from build123d import *

# Parameters (mm, degrees)
SKETCH1_R               = 13.365
BOSS_EXTRUDE1_DEPTH     = 10
SKETCH2_R               = 15
BOSS_EXTRUDE2_DEPTH     = 2
BOSS_EXTRUDE3_START     = -2
SKETCH3_R               = 15
BOSS_EXTRUDE3_DEPTH     = 2
CUT_EXTRUDE1_DEPTH      = 10
CUT_EXTRUDE1_DEPTH_BACK = 24.452078799
SKETCH4_R               = 5
SKETCH4_R_2             = 2.5


with BuildPart() as part:
    # Sketch1 → Boss-Extrude1 (new body)
    with BuildSketch(Plane(origin=(0, 0, 0), x_dir=(1, 0, 0), z_dir=(0, 1, 0))):
        with Locations(Location((0, 0, 0), (0, 0, 270))):
            Circle(SKETCH1_R)
    extrude(amount=BOSS_EXTRUDE1_DEPTH)

    # Sketch2 → Boss-Extrude2 (add)
    with BuildSketch(Plane(origin=(0, 10, 0), x_dir=(1, 0, 0), z_dir=(0, 1, 0))):
        with Locations(Location((0, 0, 0), (0, 0, 270))):
            Circle(SKETCH2_R)
    extrude(amount=-BOSS_EXTRUDE2_DEPTH)

    # Sketch3 → Boss-Extrude3 (add)
    with BuildSketch(Plane.XZ.offset(BOSS_EXTRUDE3_START)):
        with Locations(Location((0, 0, 0), (0, 0, 90))):
            Circle(SKETCH3_R)
    extrude(amount=BOSS_EXTRUDE3_DEPTH)

    # Sketch4 → Cut-Extrude1 (cut, two sides: drawn at the far end of the back side and taken through both)
    with BuildSketch(Plane.XZ.offset(-CUT_EXTRUDE1_DEPTH_BACK)):
        with Locations(Location((0, 0, 0), (0, 0, 90))):
            Circle(SKETCH4_R)
        with Locations(Location((0, 9, 0), (0, 0, 90))):
            Circle(SKETCH4_R_2)
        with Locations(Location((9, 0, 0), (0, 0, 90))):
            Circle(SKETCH4_R_2)
        with Locations(Location((0, -9, 0), (0, 0, 90))):
            Circle(SKETCH4_R_2)
        with Locations(Location((-9, 0, 0), (0, 0, 90))):
            Circle(SKETCH4_R_2)
    extrude(amount=CUT_EXTRUDE1_DEPTH + CUT_EXTRUDE1_DEPTH_BACK, mode=Mode.SUBTRACT)


solid = part.part
CAD build for the part. Positions are in the model's coordinates, mm. A direction names the side the tool comes from. Round coordinates to 2 decimals unless told otherwise and drop trailing zeros. Write each loop counter-clockwise with the first axis right and the second up, starting at its lowest first coordinate (ties: lowest second). Pieces come first, ordered by that corner, then holes. Notation, with made-up numbers: M 87,42 L 113,42 A14 cw 113,46 Z; hole C 63,61.25 d8. An arc over 180 degrees is marked long. Use a Markdown table: item, result. Add a question column.
1. 3-axis set-ups, long thin cutter, end or side, ignore diameter. For faces 1 (the face through (-4, 0, -4)), 2 (the face through (2.2, 2, -13.4)): which of +Z, -Z, +X, -X, +Y, -Y reach the whole face in a straight line?
2. Drill centre lines: probe 1 along X at (y, z) = (5.5, 0) (3 decimals); probe 2 along Z at (x, y) = (1.25, 1.5); probe 3 along Y at (x, z) = (-4.25, -13.5). Where is each one in solid material? Low to high.
3. Flat gauge pins, fed straight in: P1, Ø5, axis at y = 1.5, z = 4.5, coming from the -X side; P2, Ø4.5, axis at x = 9, z = 0, coming from the -Y side; P3, Ø4, axis at y = 4.5, z = -9.5, coming from the +X side; P4, Ø6, axis at y = 3, z = 4, coming from the -X side. Where does each tip first touch, or does it go through?
4. Slice it at A-A on z = 0. Give the cut face in (x, y) (3 decimals), then the cut area to 3 significant figures.
5. Slice it at D-D on x = -10.25. Give the cut face in (y, z).
6. Slice it at B-B on x = 0. Give the cut face in (y, z) (3 decimals), then the cut area to 3 significant figures.
7. Slice it at C-C on y = 1.25. Give the cut face in (x, z), then the cut area to 3 significant figures.
8. Pull direction X, two halves, no side cores. Call faces 3 (the face through (11.44, 5.07, -0.54)), 4 (the face through (0.66, 9.014, -14.985)), 5 (the face through (4, 10, -4)): released by +X, released by -X, zero draft, split by the parting line, or undercut.
Reply:
| question | item | result |
|---|---|---|
| 1 | face 1 | +Z, -Z, +X, -X, -Y |
| 1 | face 2 | none |
| 2 | probe 1 | x = -13.365 to -11.5, -6.5 to -5, 5 to 6.5, 11.5 to 13.365 |
| 2 | probe 2 | z = -14.95 to -11.17, -6.83 to -4.84, 4.84 to 6.83, 11.17 to 14.95 |
| 2 | probe 3 | y = 0 to 2, 8 to 10 |
| 3 | P1 | stops at x = -14.87 |
| 3 | P2 | passes through |
| 3 | P3 | stops at x = 11.06 |
| 3 | P4 | stops at x = -14.95 |
| 4 | outline | M -15,0 L -11.5,0 L -11.5,10 L -15,10 L -15,8 L -13.365,8 L -13.365,2 L -15,2 Z; M -6.5,0 L -5,0 L -5,10 L -6.5,10 Z; M 5,0 L 6.5,0 L 6.5,10 L 5,10 Z; M 11.5,0 L 15,0 L 15,2 L 13.365,2 L 13.365,8 L 15,8 L 15,10 L 11.5,10 Z |
| 4 | area | 80.4 mm^2 |
| 5 | outline | M 0,-10.95 L 2,-10.95 L 2,-8.58 L 8,-8.58 L 8,-10.95 L 10,-10.95 L 10,-2.17 L 0,-2.17 Z; M 0,2.17 L 10,2.17 L 10,10.95 L 8,10.95 L 8,8.58 L 2,8.58 L 2,10.95 L 0,10.95 Z |
| 6 | outline | M 0,-15 L 2,-15 L 2,-13.365 L 8,-13.365 L 8,-15 L 10,-15 L 10,-11.5 L 0,-11.5 Z; M 0,-6.5 L 10,-6.5 L 10,-5 L 0,-5 Z; M 0,5 L 10,5 L 10,6.5 L 0,6.5 Z; M 0,11.5 L 10,11.5 L 10,15 L 8,15 L 8,13.365 L 2,13.365 L 2,15 L 0,15 Z |
| 6 | area | 80.4 mm^2 |
| 7 | outline | C 0,0 d30; hole C -9,0 d5; hole C 0,0 d10; hole C 0,-9 d5; hole C 0,9 d5; hole C 9,0 d5 |
| 7 | area | 550 mm^2 |
| 8 | face 3 | undercut |
| 8 | face 4 | split by the parting line |
| 8 | face 5 | zero draft |
